from build123d import *

# Parameters (mm, degrees)
SKETCH1_R           = 6.942600547
BOSS_EXTRUDE1_DEPTH = 3.2004
CUT_EXTRUDE1_DEPTH  = 3.2004


with BuildPart() as part:
    # Sketch1 → Boss-Extrude1 (new body)
    with BuildSketch(Plane.XY):
        Circle(SKETCH1_R)
        Polygon((0, 3.048), (-0.315924789, 2.500802214), (-0.758006776, 2.952241475), (-0.927923651, 2.343667613), (-1.468385199, 2.670982761), (-1.481617658, 2.039271757), (-2.086499579, 2.221896376), (-1.942216178, 1.606740957), (-2.573511517, 1.633200071), (-2.280778112, 1.073252713), (-2.898820262, 0.941883799), (-2.47603037, 0.472328054), (-3.041985468, 0.191385504), (-2.515704533, -0.158274714), (-2.99401154, -0.571138247), (-2.397307729, -0.778932499), (-2.757912856, -1.297775281), (-2.128279263, -1.350647091), (-2.348524364, -1.942868321), (-1.725523184, -1.837495558), (-1.791569449, -2.465883799), (-1.214346137, -2.208887422), (-1.122043637, -2.833958729), (-0.626867256, -2.441486766), (-0.382015696, -3.02396561), (0, -2.520678517), (0.382015696, -3.02396561), (0.626867256, -2.441486766), (1.122043637, -2.833958729), (1.214346137, -2.208887422), (1.791569449, -2.465883799), (1.725523184, -1.837495558), (2.348524364, -1.942868321), (2.128279263, -1.350647091), (2.757912856, -1.297775281), (2.397307729, -0.778932499), (2.99401154, -0.571138247), (2.515704533, -0.158274714), (3.041985468, 0.191385504), (2.47603037, 0.472328054), (2.898820262, 0.941883799), (2.280778112, 1.073252713), (2.573511517, 1.633200071), (1.942216178, 1.606740957), (2.086499579, 2.221896376), (1.481617658, 2.039271757), (1.468385199, 2.670982761), (0.927923651, 2.343667613), (0.758006776, 2.952241475), (0.315924789, 2.500802214), align=None, mode=Mode.SUBTRACT)
    extrude(amount=BOSS_EXTRUDE1_DEPTH)

    # Sketch2 → Cut-Extrude1 (cut)
    with BuildSketch(Plane.XY.offset(3.2004)):
        with BuildLine():
            Line((-1.297184474, 6.820338319), (-0.259835526, 4.836738163))
            ThreePointArc((-0.259835526, 4.836738163), (0, 4.679400627), (0.259835526, 4.836738163))
            Line((0.259835526, 4.836738163), (1.297184474, 6.820338319))
            ThreePointArc((1.297184474, 6.820338319), (0, 6.942600547), (-1.297184474, 6.820338319))
        make_face()
        with BuildLine():
            Line((2.643393248, 4.058820358), (4.533563867, 5.25799401))
            ThreePointArc((4.533563867, 5.25799401), (3.471300273, 6.012468442), (2.286774452, 6.555178484))
            Line((2.286774452, 6.555178484), (2.193344915, 4.318655884))
            ThreePointArc((2.193344915, 4.318655884), (2.339700314, 4.052479818), (2.643393248, 4.058820358))
        make_face()
        with BuildLine():
            Line((4.318655884, 2.193344915), (6.555178484, 2.286774452))
            ThreePointArc((6.555178484, 2.286774452), (6.012468442, 3.471300273), (5.25799401, 4.533563867))
            Line((5.25799401, 4.533563867), (4.058820358, 2.643393248))
            ThreePointArc((4.058820358, 2.643393248), (4.052479818, 2.339700314), (4.318655884, 2.193344915))
        make_face()
        with BuildLine():
            Line((4.836738163, -0.259835526), (6.820338319, -1.297184474))
            ThreePointArc((6.820338319, -1.297184474), (6.942600547, 0), (6.820338319, 1.297184474))
            Line((6.820338319, 1.297184474), (4.836738163, 0.259835526))
            ThreePointArc((4.836738163, 0.259835526), (4.679400627, 0), (4.836738163, -0.259835526))
        make_face()
        with BuildLine():
            Line((4.058820358, -2.643393248), (5.25799401, -4.533563867))
            ThreePointArc((5.25799401, -4.533563867), (6.012468442, -3.471300273), (6.555178484, -2.286774452))
            Line((6.555178484, -2.286774452), (4.318655884, -2.193344915))
            ThreePointArc((4.318655884, -2.193344915), (4.052479818, -2.339700314), (4.058820358, -2.643393248))
        make_face()
        with BuildLine():
            Line((2.193344915, -4.318655884), (2.286774452, -6.555178484))
            ThreePointArc((2.286774452, -6.555178484), (3.471300273, -6.012468442), (4.533563867, -5.25799401))
            Line((4.533563867, -5.25799401), (2.643393248, -4.058820358))
            ThreePointArc((2.643393248, -4.058820358), (2.339700314, -4.052479818), (2.193344915, -4.318655884))
        make_face()
        with BuildLine():
            Line((-0.259835526, -4.836738163), (-1.297184474, -6.820338319))
            ThreePointArc((-1.297184474, -6.820338319), (0, -6.942600547), (1.297184474, -6.820338319))
            Line((1.297184474, -6.820338319), (0.259835526, -4.836738163))
            ThreePointArc((0.259835526, -4.836738163), (0, -4.679400627), (-0.259835526, -4.836738163))
        make_face()
        with BuildLine():
            Line((-2.643393248, -4.058820358), (-4.533563867, -5.25799401))
            ThreePointArc((-4.533563867, -5.25799401), (-3.471300273, -6.012468442), (-2.286774452, -6.555178484))
            Line((-2.286774452, -6.555178484), (-2.193344915, -4.318655884))
            ThreePointArc((-2.193344915, -4.318655884), (-2.339700314, -4.052479818), (-2.643393248, -4.058820358))
        make_face()
        with BuildLine():
            Line((-4.318655884, -2.193344915), (-6.555178484, -2.286774452))
            ThreePointArc((-6.555178484, -2.286774452), (-6.012468442, -3.471300273), (-5.25799401, -4.533563867))
            Line((-5.25799401, -4.533563867), (-4.058820358, -2.643393248))
            ThreePointArc((-4.058820358, -2.643393248), (-4.052479818, -2.339700314), (-4.318655884, -2.193344915))
        make_face()
        with BuildLine():
            Line((-4.836738163, 0.259835526), (-6.820338319, 1.297184474))
            ThreePointArc((-6.820338319, 1.297184474), (-6.942600547, 0), (-6.820338319, -1.297184474))
            Line((-6.820338319, -1.297184474), (-4.836738163, -0.259835526))
            ThreePointArc((-4.836738163, -0.259835526), (-4.679400627, 0), (-4.836738163, 0.259835526))
        make_face()
        with BuildLine():
            Line((-4.058820358, 2.643393248), (-5.25799401, 4.533563867))
            ThreePointArc((-5.25799401, 4.533563867), (-6.012468442, 3.471300273), (-6.555178484, 2.286774452))
            Line((-6.555178484, 2.286774452), (-4.318655884, 2.193344915))
            ThreePointArc((-4.318655884, 2.193344915), (-4.052479818, 2.339700314), (-4.058820358, 2.643393248))
        make_face()
        with BuildLine():
            Line((-2.193344915, 4.318655884), (-2.286774452, 6.555178484))
            ThreePointArc((-2.286774452, 6.555178484), (-3.471300273, 6.012468442), (-4.533563867, 5.25799401))
            Line((-4.533563867, 5.25799401), (-2.643393248, 4.058820358))
            ThreePointArc((-2.643393248, 4.058820358), (-2.339700314, 4.052479818), (-2.193344915, 4.318655884))
        make_face()
    extrude(amount=-CUT_EXTRUDE1_DEPTH, mode=Mode.SUBTRACT)


solid = part.part
Verification items for the finished model (mm, model axes). A direction names the side the tool comes from. Coordinates: 2 decimals unless noted, no trailing zeros. Write each loop counter-clockwise with the first axis right and the second up, starting at its lowest first coordinate (ties: lowest second). Pieces come first, ordered by that corner, then holes. Notation, with made-up numbers: M -28,40.5 L -17,40.5 A30 ccw -17,69.5 Z; hole C -3,12 d6. An arc over 180 degrees is marked long. Use a Markdown table: item, result.
Q1. Sectioned sample at A-A, the plane y = 0. Record the boundary of the cut face in (x, z), plus the area to 3 significant figures.
Reply:
| item | result |
|---|---|
| outline | M -4.68,0 L -2.75,0 L -2.75,3.2 L -4.68,3.2 Z; M 2.75,0 L 4.68,0 L 4.68,3.2 L 2.75,3.2 Z |
| area | 12.3 mm² |
Q2. Go/stop test with flat-tipped pins: P1, Ø1.5, axis at x = -0.5, y = 1.5, coming from the +Z side (1 decimal); P2, Ø1, axis at y = 3.5, z = 1.5, coming from the +X side. Record where each tip stops, or that it passes through.
Reply:
| item | result |
|---|---|
| P1 | passes through |
| P2 | stops at x = 4.92 |
Q3. Sectioned sample at B-B, the plane y = -3.75. Record the boundary of the cut face in (x, z), plus the area to 3 significant figures.
Reply:
| item | result |
|---|---|
| outline | M -4.76,0 L 4.76,0 L 4.76,3.2 L -4.76,3.2 Z |
| area | 30.5 mm² |
Q4. Set-up check for faces 1 (the face through (4.667, 3.602, 1.623)), 2 (the face through (0.786, -5.842, 1.623)), 3 (the face through (-4.667, -3.602, 1.623)): record each of +Z, -Z, +X, -X, +Y, -Y from which the full face is reachable in a straight line by a thin tool's end or side.
Reply:
| item | result |
|---|---|
| face 1 | +Z, -Z, +X |
| face 2 | +Z, -Z, -Y |
| face 3 | +Z, -Z, -X |
Q5. Draft check along Y on faces 4 (the face through (0, -3, 3.2)), 5 (the face through (5.81, -0.77, 1.62)), 6 (the face through (-3.575, -4.65, 1.623)). Enter one of: +Y half, -Y half, draft (parallel to the pull), parting line (faces both ways), or undercut.
Reply:
| item | result |
|---|---|
| face 4 | draft |
| face 5 | undercut |
| face 6 | -Y half |
Q6. Thickness scan on line 1 (X direction, y = 0, z = 1.35); line 2 (Y direction, x = -5, z = 0.9); line 3 (X direction, y = -4.75, z = 2.45). Record the ranges inside material, lowest first.
Reply:
| item | result |
|---|---|
| line 1 | x = -4.68 to -2.75, 2.75 to 4.68 |
| line 2 | y = -4.82 to -4.13, -2.22 to -0.35, 0.35 to 2.22, 4.13 to 4.82 |
| line 3 | x = -5.06 to -3.73, -2.21 to -0.19, 0.19 to 2.21, 3.73 to 5.06 |
